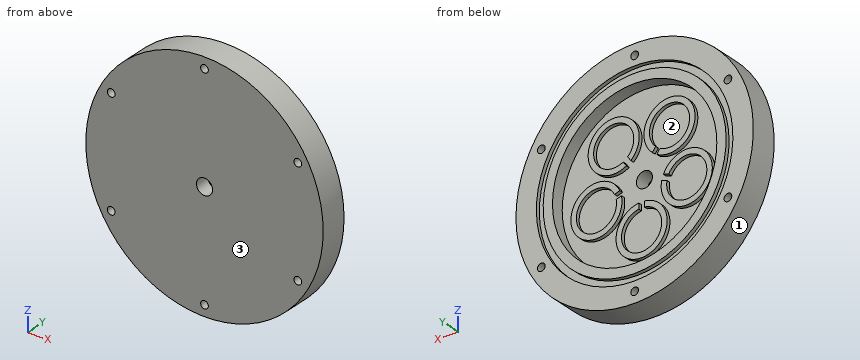
```python
from build123d import *

# Parameters (mm, degrees)
CROQUIS2_R              = 65
SALIENTE_EXTRUIR1_DEPTH = 15
CROQUIS2_3_R            = 45
CORTAR_EXTRUIR1_DEPTH   = 7
TALADRO_ROSCADO_G1_81_D = 8.8
CROQUIS3_R              = 14
CROQUIS3_R_2            = 11
SALIENTE_EXTRUIR3_DEPTH = 2
CORTAR_EXTRUIR3_DEPTH   = 8
MATRIZC1_COUNT          = 5
CROQUIS7_W              = 3.7
CROQUIS7_H              = 4.2
TALADRO_ROSCADO_M51_D   = 4.2
MATRIZC2_COUNT          = 6


with BuildPart() as part:
    # Croquis2 → Saliente-Extruir1 (new body)
    with BuildSketch(Plane(origin=(0, 0, 0), x_dir=(1, 0, 0), z_dir=(0, 1, 0))):
        Circle(CROQUIS2_R)
    extrude(amount=-SALIENTE_EXTRUIR1_DEPTH)

    # Croquis2_3 → Cortar-Extruir1 (cut)
    with BuildSketch(Plane(origin=(0, 0, 0), x_dir=(1, 0, 0), z_dir=(0, 1, 0))):
        Circle(CROQUIS2_3_R)
    extrude(amount=-CORTAR_EXTRUIR1_DEPTH, mode=Mode.SUBTRACT)

    # Taladro roscado G1_81 (through all)
    with Locations(Plane(origin=(0, -15, 0), x_dir=(-1, 0, 0), z_dir=(0, -1, 0))):
        with Locations((0, 0)):
            Hole(TALADRO_ROSCADO_G1_81_D / 2)

    # Croquis3 → Saliente-Extruir3 (add)
    with BuildSketch(Plane(origin=(0, -7, 0), x_dir=(1, 0, 0), z_dir=(0, 1, 0))):
        with Locations((0, 26)):
            Circle(CROQUIS3_R)
        with Locations((0, 26)):
            Circle(CROQUIS3_R_2, mode=Mode.SUBTRACT)
    saliente_extruir3 = extrude(amount=SALIENTE_EXTRUIR3_DEPTH)

    # Croquis6 → Cortar-Extruir3 (cut, through all)
    with BuildSketch(Plane(origin=(0, -7, 0), x_dir=(1, 0, 0), z_dir=(0, 1, 0))):
        with BuildLine():
            Line((1.5, 26), (1.5, 4.4))
            ThreePointArc((1.5, 4.4), (0, 2.9), (-1.5, 4.4))
            Line((-1.5, 4.4), (-1.5, 26))
            ThreePointArc((-1.5, 26), (0, 27.5), (1.5, 26))
        make_face()
    cortar_extruir3 = extrude(amount=CORTAR_EXTRUIR3_DEPTH, mode=Mode.SUBTRACT)

    # MatrizC1: Saliente-Extruir3, Cortar-Extruir3 ×5 about axis
    matrizc1_axis = Axis((0, 0, 0), (0, 1, 0))
    for i in range(1, MATRIZC1_COUNT):
        add(saliente_extruir3.rotate(matrizc1_axis, i * 360 / MATRIZC1_COUNT))
        add(cortar_extruir3.rotate(matrizc1_axis, i * 360 / MATRIZC1_COUNT), mode=Mode.SUBTRACT)

    # Croquis7 → Cortar-Revoluci_n1 (revolve, cut)
    with BuildSketch(Plane(origin=(0, 0, 0), x_dir=(0, 0, -1), z_dir=(1, 0, 0))):
        with Locations((51.945, 0)):
            Rectangle(CROQUIS7_W, CROQUIS7_H)
    revolve(axis=Axis((0, 0, 0), (0, -1, 0)), mode=Mode.SUBTRACT)

    # Taladro roscado M51 (through all)
    with Locations(Plane(origin=(0, 0, 0), x_dir=(1, 0, 0), z_dir=(0, 1, 0))):
        with Locations((0, 59)):
            taladro_roscado_m51 = Hole(TALADRO_ROSCADO_M51_D / 2)

    # MatrizC2: Taladro roscado M51 ×6 about axis
    matrizc2_axis = Axis((0, 0, 0), (0, 1, 0))
    for i in range(1, MATRIZC2_COUNT):
        add(taladro_roscado_m51.rotate(matrizc2_axis, i * 360 / MATRIZC2_COUNT), mode=Mode.SUBTRACT)


solid = part.part
```
Can you work these out from the model? Positions are in its coordinate system, mm. Face numbers are marked on the shaded views. Round coordinates to 2 decimals unless told otherwise and drop trailing zeros. Loops run counter-clockwise (first coordinate to the right, second up) from the corner with the lowest first, then second, coordinate; pieces in that order, holes last. Notation, with made-up numbers: M 47,-24 L 81,-24 A23 cw 81,14 Z; hole C 48.25,25 d4. An arc over 180 degrees is marked long. Answer in a Markdown table with one row per item.
1. If we section it at A-A, the plane z = 59: Please give me the cut outline in (x, y), plus the area to 3 significant figures.
Established:
| item | result |
|---|---|
| outline | M -27.28,-15 L -2.1,-15 L -2.1,0 L -27.28,0 Z; M 2.1,-15 L 27.28,-15 L 27.28,0 L 2.1,0 Z |
| area | 755 mm² |
2. Please list where these lines run through material, in increasing order: line 1 (X direction, y = -8, z = -29); line 2 (X direction, y = -1.25, z = -18); line 3 (Z direction, x = 5.5, y = -6). Write a range as from..to.
Established:
| item | result |
|---|---|
| line 1 | -58.17..-53.14, -49.06..49.06, 53.14..58.17 |
| line 2 | -62.46..-50.69, -46.75..-41.24, 41.24..46.75, 50.69..62.46 |
| line 3 | -64.77..-44.66, -38.87..-35.53, -16.47..-13.13, 11.02..16, 26.06..31.05, 44.66..64.77 |
3. Thinking about a two-plate mould opening in Z: for the marked faces 1, 2 and 3, which applies, pulls with the +Z half, pulls with the -Z half, needs draft (parallel to the pull), parting line crosses it, or undercut?
Established:
| item | result |
|---|---|
| face 1 | parting line crosses it |
| face 2 | undercut |
| face 3 | needs draft |
4. I'm going to push flat-ended pins straight in: pin 1 Ø6 at (x, y) = (-28.5, -10.5) entering from -Z; pin 2 Ø0.6 at (y, z) = (-5.5, -13.5) entering from +X; pin 3 Ø14 at (x, z) = (4, -22) entering from +Y; pin 4 Ø4 at (x, z) = (0, 59) entering from -Y. Where does each tip first touch, or does it pass through?
Established:
| item | result |
|---|---|
| pin 1 | z = -59.79 |
| pin 2 | x = 63.65 |
| pin 3 | y = -5 |
| pin 4 | through |
5. If we section it at C-C, the plane z = -29.5: Give the number of separate pieces and of enclosed holes in the cut face, plus the area to 3 significant figures.
Established:
| item | result |
|---|---|
| separate pieces | 3 |
| enclosed holes | 0 |
| area | 1,130 mm² |
6. If we section it at B-B, the plane y = -12.5: Please give me the cut outline in (x, z).
Established:
| item | result |
|---|---|
| outline | C 0,0 d130; hole C -51.1,-29.5 d4.2; hole C -51.1,29.5 d4.2; hole C 0,0 d8.8; hole C 0,-59 d4.2; hole C 0,59 d4.2; hole C 51.1,-29.5 d4.2; hole C 51.1,29.5 d4.2 |
